Source: CAD feature listing. Evaluate the final solid. Frame: model axes, mm. Give positions to 0.01 mm unless a question says otherwise; leave off trailing zeros. Order: outer loops, then holes, each group sorted by start corner. A loop starts at its lowest first (then second) coordinate and runs counter-clockwise, first axis right, second up. Notation, with made-up numbers: (-4.75, 55) - (54.25, 55) arc R17 cw to (54.25, 78) - close; hole circle Ø1 at (75, 23.5). An arc over 180 degrees is marked (long way). Use CSV: the item, a comma, the result in double quotes.
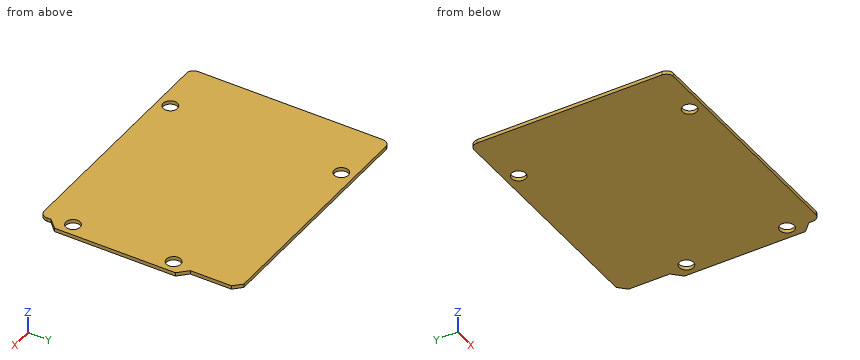
```python
from build123d import *

# Parameters (mm, degrees)
SKETCH_R      = 2
EXTRUDE_DEPTH = 1


with BuildPart() as part:
    # Sketch → Extrude (new body)
    with BuildSketch(Plane.XY):
        with BuildLine():
            Line((1, 54.65), (65.264214, 54.65))
            Line((65.264214, 54.65), (67.4, 52.514214))
            Line((67.4, 52.514214), (67.4, 41.014214))
            Line((67.4, 41.014214), (69.95, 38.464214))
            Line((69.95, 38.464214), (69.95, 4.685786))
            Line((69.95, 4.685786), (67.4, 2.135786))
            Line((67.4, 2.135786), (67.4, 1))
            ThreePointArc((65.4, -1), (66.814214, -0.414214), (67.4, 1))
            Line((65.4, -1), (1, -1))
            ThreePointArc((-1, 1), (-0.414214, -0.414214), (1, -1))
            Line((-1, 1), (-1, 52.65))
            ThreePointArc((1, 54.65), (-0.414214, 54.064214), (-1, 52.65))
        make_face()
        with Locations((15.334135, 51.082933)):
            Circle(SKETCH_R, mode=Mode.SUBTRACT)
        with Locations((66.409951, 35.749834)):
            Circle(SKETCH_R, mode=Mode.SUBTRACT)
        with Locations((66.413926, 7.668398)):
            Circle(SKETCH_R, mode=Mode.SUBTRACT)
        with Locations((14.05247, 2.556984)):
            Circle(SKETCH_R, mode=Mode.SUBTRACT)
    extrude(amount=EXTRUDE_DEPTH)


solid = part.part
```
Item 1: First-contact query: pin 1 (3.5 mm diameter, centred on x = 66.41, y = 7.67, fed in from -Z). Flat tip, straight axial feed; report the tip coordinate or a pass-through.
Filled in:
pin 1,"passes through"
Item 2: Section A-A on y = 36.5. Return the cut outline in (x, z).
Filled in:
outline,"(-1, 0) - (64.56, 0) - (64.56, 1) - (-1, 1) - close; (68.26, 0) - (69.95, 0) - (69.95, 1) - (68.26, 1) - close"
Item 3: Section B-B on z = 0.35. Return the cut outline in (x, y).
Filled in:
outline,"(-1, 1) arc R2 ccw to (1, -1) - (65.4, -1) arc R2 ccw to (67.4, 1) - (67.4, 2.14) - (69.95, 4.69) - (69.95, 38.46) - (67.4, 41.01) - (67.4, 52.51) - (65.26, 54.65) - (1, 54.65) arc R2 ccw to (-1, 52.65) - close; hole circle Ø4 at (14.05, 2.56); hole circle Ø4 at (15.33, 51.08); hole circle Ø4 at (66.41, 7.67); hole circle Ø4 at (66.41, 35.75)"
Item 4: Material intervals for line 1 (X direction, y = 7.5, z = 0.95); line 2 (X direction, y = 4, z = 0.4); line 3 (X direction, y = 45, z = 0.9), sorted ascending. Write a range as from..to.
Filled in:
line 1,"x = -1..64.42, 68.41..69.95"
line 2,"x = -1..12.67, 15.44..69.26"
line 3,"x = -1..67.4"
